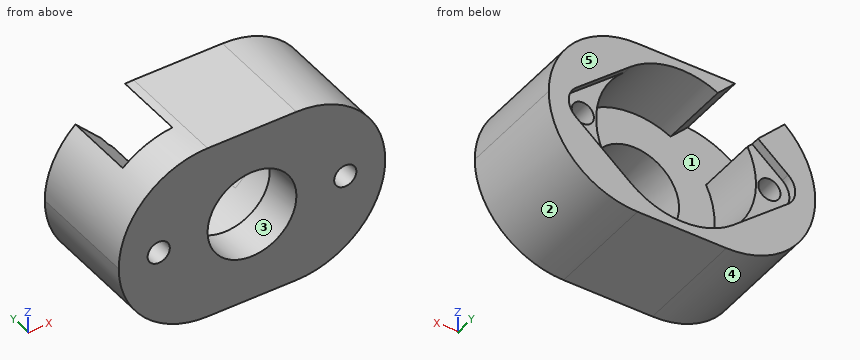
Autodesk Fusion 360 part; units mm, degrees
box "BoxPrimitive1" add length 40 width 60 height 25 placed x (0, 0, -1) y (-1, 0, 0) z (0, 1, 0) at (30, 0, 20)
cylinder "CylinderPrimitive1" cut diameter 36 height -16 placed x (1, 0, 0) y (0, 0, -1) z (0, 1, 0) at (0, 25, 0)
hole "Hole1" at (0, 9, 0) direction (0, -1, 0) diameter 20 depth 17 tip angle 118
sketch "Sketch4" plane through (0, 25, 0) normal (0, 1, 0) x (-1, 0, 0)
  circle A0 centre (0, 0) radius 18
  line L0 (-30, -20) -> (30, -20)
  line L1 (30, -20) -> (30, 20)
  line L2 (30, 20) -> (-30, 20)
  line L3 (-30, 20) -> (-30, -20)
  arc A1 (23.8929, -3.4469) -> (23.8929, 3.4469) centre (21, 0) ccw
  arc A2 (-23.8929, 3.4469) -> (-23.8929, -3.4469) centre (-21, 0) ccw
  arc A3 (-11.5714, -13.7877) -> (11.5714, -13.7877) centre (0, 0) ccw
  arc A4 (11.5714, 13.7877) -> (-11.5714, 13.7877) centre (0, 0) ccw
  line L4 (23.8929, -3.4469) -> (11.5714, -13.7877)
  line L5 (-11.5714, -13.7877) -> (-23.8929, -3.4469)
  line L6 (-23.8929, 3.4469) -> (-11.5714, 13.7877)
  line L7 (11.5714, 13.7877) -> (23.8929, 3.4469)
  dimension "d11" = 4.5
  dimension "d12" = 4.5
  dimension "d13" = 21
  dimension "d14" = 21
extrude "Extrude1" cut sketch "Sketch4" against normal blind 2 contours A0 A1 L4 L7 | A0 A2 L5 L6
hole "Hole2" at (-21, 23, 0) direction (0, -1, 0) diameter 5 end through all
hole "Hole3" at (21, 23, 0) direction (0, -1, 0) diameter 5 end through all
fillet "Fillet1" radius 20 1 edges at (-30, 12.5, 20)
fillet "Fillet1" radius 20 3 edges at (30, 12.5, 20) (30, 12.5, -20) (-30, 12.5, -20)
sketch "Sketch5" plane through (0, 25, 0) normal (0, 1, 0) x (-1, 0, 0)
  arc A0 (10, -20) -> (10, 20) centre (10, 0) ccw
  line L0 (10, 20) -> (-10, 20)
  arc A1 (-10, 20) -> (-10, -20) centre (-10, 0) ccw
  line L1 (-10, -20) -> (10, -20)
  line L2 (23.8929, -3.4469) -> (11.5714, -13.7877)
  arc A2 (-11.5714, -13.7877) -> (11.5714, -13.7877) centre (0, 0) ccw
  line L3 (-11.5714, -13.7877) -> (-23.8929, -3.4469)
  arc A3 (-23.8929, 3.4469) -> (-23.8929, -3.4469) centre (-21, 0) ccw
  line L4 (-23.8929, 3.4469) -> (-11.5714, 13.7877)
  arc A4 (11.5714, 13.7877) -> (-11.5714, 13.7877) centre (0, 0) ccw
  line L5 (11.5714, 13.7877) -> (23.8929, 3.4469)
  arc A5 (23.8929, -3.4469) -> (23.8929, 3.4469) centre (21, 0) ccw
  line L6 (8, 0) -> (0, 8)
  line L7 (0, 8) -> (20.2173, 28.2173)
  line L8 (20.2173, 28.2173) -> (28.2173, 20.2173)
  line L9 (28.2173, 20.2173) -> (8, 0)
  dimension "d25" = 8
  dimension "d26" = 8
extrude "Extrude2" cut sketch "Sketch5" against normal blind 16 contours A0 A4 L5 L7 L9 | A0 L7 L8 L9 | A4 L5 L6 L7 L9
equation "d13 = ( 42 / 2 ) * 1 mm"
equation "d14 = ( 42 / 2 ) * 1 mm"
Can you work these out from the model? Positions are in its coordinate system, mm. Face numbers are marked on the shaded views. A direction names the side the tool comes from. Coordinates: 2 decimals unless noted, no trailing zeros. Loops run counter-clockwise (first coordinate to the right, second up) from the corner with the lowest first, then second, coordinate; pieces in that order, holes last. Notation, with made-up numbers: (34.25, -1.75) - (51.25, -1.75) arc R18 ccw to (51.25, 21.25) - close; hole circle Ø2 at (18.5, -16). An arc over 180 degrees is marked (long way). Use a Markdown table: item, result.
Item 1: I want a section at B-B on x = 21. Please give me the cut outline in (y, z).
Numbers:
| item | result |
|---|---|
| outline | (0, -16.71) - (25, -16.71) - (25, -5.87) - (23, -5.87) - (23, -2.5) - (0, -2.5) - close; (0, 2.5) - (23, 2.5) - (23, 5.87) - (25, 5.87) - (25, 16.71) - (0, 16.71) - close |
Item 2: I want a section at D-D on z = 6.5. Please give me the cut outline in (x, y) (3 decimals).
Numbers:
| item | result |
|---|---|
| outline | (-28.915, 0) - (-7.599, 0) - (-7.599, 9) - (-16.785, 9) - (-16.785, 23) - (-20.255, 23) - (-20.255, 25) - (-28.915, 25) - close; (7.599, 0) - (28.915, 0) - (28.915, 25) - (20.255, 25) - (20.255, 23) - (16.785, 23) - (16.785, 9) - (7.599, 9) - close |
Item 3: Will these pins go through, and if not, where does the flat tip stop? pin 1 (6 mm diameter, centred on y = 11, z = 11, fed in from +X); pin 2 (1 mm diameter, centred on y = 12.5, z = 9, fed in from +X); pin 3 (3 mm diameter, centred on x = -24, y = 22, fed in from -Z).
Numbers:
| item | result |
|---|---|
| pin 1 | stops at x = 28.33 |
| pin 2 | stops at x = 28.11 |
| pin 3 | stops at z = -15.61 |
Item 4: We'd pull the mould along Z, two halves only. Please class the marked faces 3, 4 and 5: released by +Z, released by -Z, zero draft, split by the parting line, or undercut.
Numbers:
| item | result |
|---|---|
| face 3 | undercut |
| face 4 | released by -Z |
| face 5 | zero draft |
Item 5: I want a section at A-A on y = 5.5. Give the number of separate pieces and of enclosed holes in the cut face, and give its area (3 significant figures).
Numbers:
| item | result |
|---|---|
| separate pieces | 1 |
| enclosed holes | 3 |
| area | 1,700 mm2 |
Item 6: If I drill on probe 1 along X at (y, z) = (3.25, 0); probe 2 along Z at (x, y) = (0, 4.75); probe 3 along X at (y, z) = (13.75, -9), over which ranges is the centre line in solid material (lowest first)? Write a range as from..to.
Numbers:
| item | result |
|---|---|
| probe 1 | x = -30..-23.5, -18.5..-10, 10..18.5, 23.5..30 |
| probe 2 | z = -20..-10, 10..20 |
| probe 3 | x = -27.86..-15.59, 15.59..27.86 |
Item 7: For the marked faces 1 and 2, which set-ups out of +Z, -Z, +X, -X, +Y, -Y let a thin tool reach every point of the face, with its end or its side?
Numbers:
| item | result |
|---|---|
| face 1 | +Y |
| face 2 | -Z, +X, +Y, -Y |
